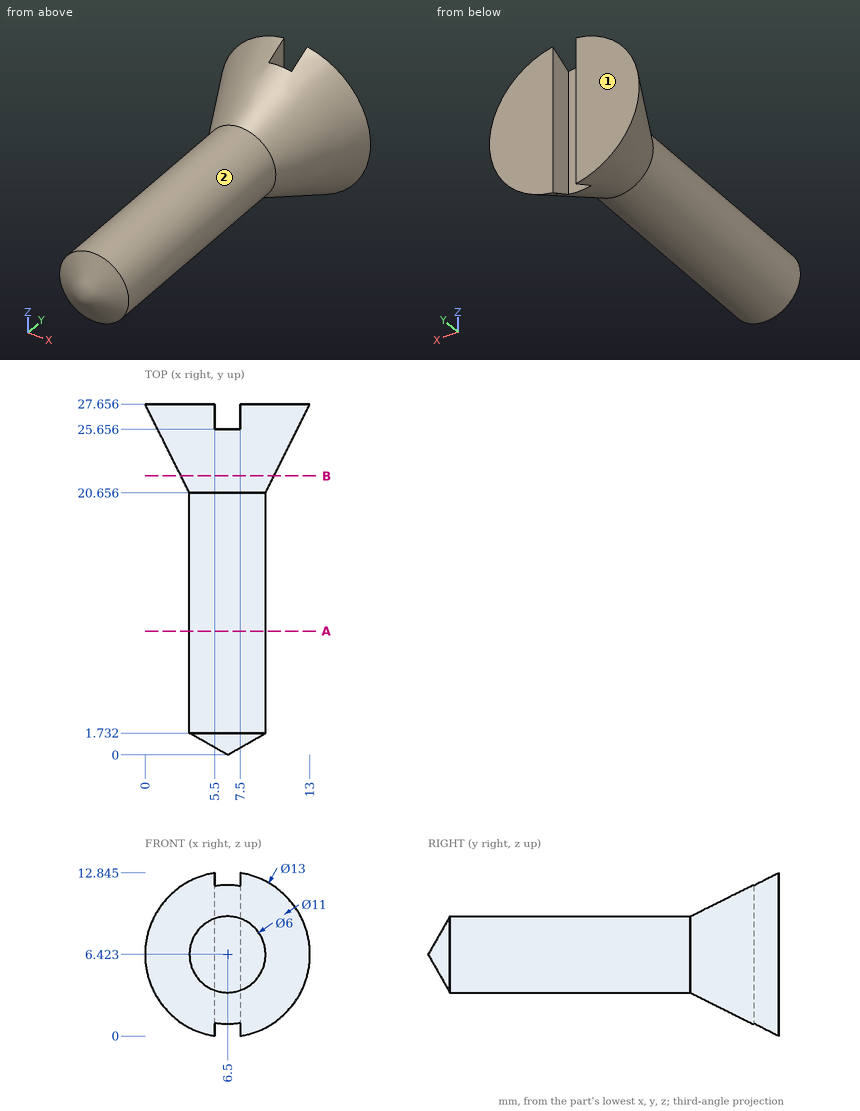
Geometry check sheet. Reference: drawing and pictorial views, mm from the part's lowest x, y, z. A direction names the side the tool comes from. Give positions to 0.01 mm unless a question says otherwise; leave off trailing zeros. Loops run counter-clockwise (first coordinate to the right, second up) from the corner with the lowest first, then second, coordinate; pieces in that order, holes last. Notation, with made-up numbers: (40, -5) -> (62, -5) arc R31 cw to (62, 30) -> close; hole circle Ø9 at (-39, -15). An arc over 180 degrees is marked (long way). Answer in a Markdown table with one row per item. Add a question column.
1) Set-up check for the marked faces 1 and 2: record each of +Z, -Z, +X, -X, +Y, -Y from which the full face is reachable in a straight line by a thin tool's end or side.
2) Cross-section at A-A on y = 9.75. Record the boundary of the cut face in (x, z).
3) Cross-section at B-B on y = 22. Record the boundary of the cut face in (x, z) (1 decimal).
4) Material ranges on probe 1 along Y at (x, z) = (4.5, 7) (1 decimal); probe 2 along X at (y, z) = (2, 8.5) (1 decimal); probe 3 along Z at (x, y) = (7, 7.75) (1 decimal), recorded low to high. Write a range as from..to.
5) Gauge pin test, flat ends, axial feed: P1, Ø0.6, axis at y = 26.5, z = 3, coming from the +X side; P2, Ø1.5, axis at x = 9, y = 3.5, coming from the +Z side; P3, Ø1, axis at x = 6.5, z = 4.5, coming from the +Y side. Record the tip position at first contact, or that the pin passes through.
Outcome:
| question | item | result |
|---|---|---|
| 1 | face 1 | +Z, -Z, +X, -X, +Y |
| 1 | face 2 | -Y |
| 2 | outline | circle Ø6 at (6.5, 6.42) |
| 3 | outline | circle Ø7.3 at (6.5, 6.4) |
| 4 | probe 1 | y = 1.2..27.7 |
| 4 | probe 2 | x = 4.3..8.7 |
| 4 | probe 3 | z = 3.5..9.4 |
| 5 | P1 | stops at x = 11.6 |
| 5 | P2 | stops at z = 8.86 |
| 5 | P3 | stops at y = 25.66 |
